Geometry: final body of the model. Coordinates: model frame, mm. A direction names the side the tool comes from. Give positions to 0.01 mm unless a question says otherwise; leave off trailing zeros. Loops run counter-clockwise (first coordinate to the right, second up) from the corner with the lowest first, then second, coordinate; pieces in that order, holes last. Notation, with made-up numbers: (32, 37) - (55, 37) arc R9 ccw to (55, 47) - close; hole circle Ø8 at (-8, 80). An arc over 180 degrees is marked (long way). Use one line per item in the form item = value.
```python
from build123d import *

# Parameters (mm, degrees)
PAD_DEPTH       = 5.3
SKETCH001_R     = 4.15
POCKET_DEPTH    = 2.3
SKETCH002_R     = 2.05
POCKET001_DEPTH = 3.001
FILLET_R        = 2.6
SKETCH003_R     = 1.625
POCKET002_DEPTH = 12.001
FILLET001_R     = 0.9
FILLET002_R     = 5
SKETCH004_R     = 2.05
POCKET003_DEPTH = 5.301
FILLET003_R     = 0.99
CHAMFER_SIZE    = 0.5
SKETCH005_W     = 0.5
SKETCH005_H     = 0.8
POCKET004_DEPTH = 4
CHAMFER001_SIZE = 0.6


with BuildPart() as part:
    # Sketch → Pad (new body)
    with BuildSketch(Plane.XY):
        Polygon((0, 5.5), (-45, 5.5), (-45, -5.5), (0, -5.5), (0, -6.5), (35, -6.5), (35, 6.5), (0, 6.5), align=None)
    extrude(amount=PAD_DEPTH)

    # Sketch001 (on Face10 of Pad) → Pocket (cut)
    with BuildSketch(Plane.XY.offset(5.3)):
        with Locations((-6, 0)):
            Circle(SKETCH001_R)
    extrude(amount=-POCKET_DEPTH, mode=Mode.SUBTRACT)

    # Sketch002 (on Face12 of Pocket) → Pocket001 (cut, through all)
    with BuildSketch(Plane.XY.offset(3)):
        with Locations((-6, 0)):
            Circle(SKETCH002_R)
    extrude(amount=-POCKET001_DEPTH, mode=Mode.SUBTRACT)

    # Fillet
    fillet_edges = [part.edges().sort_by_distance(p)[0] for p in [
        (-45, 0, 5.3),
        (-45, 0, 0),
    ]]
    fillet(fillet_edges, radius=FILLET_R)

    # Sketch003 (on Face1 of Fillet) → Pocket002 (cut, through all)
    with BuildSketch(Plane(origin=(0, 5.5, 0), x_dir=(-1, 0, 0), z_dir=(0, 1, 0))):
        with Locations((42, 2.65)):
            Circle(SKETCH003_R)
    extrude(amount=-POCKET002_DEPTH, mode=Mode.SUBTRACT)

    # Fillet001
    fillet001_edges = [part.edges().sort_by_distance(p)[0] for p in [
        (0, 6.5, 2.65),
        (0, -6.5, 2.65),
    ]]
    fillet(fillet001_edges, radius=FILLET001_R)

    # Fillet002
    fillet002_edges = [part.edges().sort_by_distance(p)[0] for p in [
        (35, 6.5, 2.65),
        (35, -6.5, 2.65),
    ]]
    fillet(fillet002_edges, radius=FILLET002_R)

    # Sketch004 (on Face15 of Fillet002) → Pocket003 (cut, through all)
    with BuildSketch(Plane.XY.offset(5.3)):
        with Locations((-15, 0)):
            Circle(SKETCH004_R)
    extrude(amount=-POCKET003_DEPTH, mode=Mode.SUBTRACT)

    # Fillet003
    fillet003_edges = [part.edges().sort_by_distance(p)[0] for p in [
        (0.263604, -6.236396, 5.3),
        (15.45, -6.5, 5.3),
        (33.535534, -5.035534, 5.3),
        (35, 0, 5.3),
        (33.535534, 5.035534, 5.3),
        (15.45, 6.5, 5.3),
        (0.263604, 6.236396, 5.3),
        (0.263604, 6.236396, 0),
        (15.45, 6.5, 0),
        (33.535534, 5.035534, 0),
        (35, 0, 0),
        (33.535534, -5.035534, 0),
        (15.45, -6.5, 0),
    ]]
    fillet(fillet003_edges, radius=FILLET003_R)

    # Chamfer
    chamfer_edges = [part.edges().sort_by_distance(p)[0] for p in [
        (-17.05, 0, 0),
        (-8.05, 0, 0),
    ]]
    chamfer(chamfer_edges, length=CHAMFER_SIZE)

    # Sketch005 (on Face1 of Chamfer) → Pocket004 (cut)
    with BuildSketch(Plane(origin=(0, 0, 0), x_dir=(1, 0, 0), z_dir=(0, 0, -1))):
        with Locations((-17.15, 0)):
            Rectangle(SKETCH005_W, SKETCH005_H)
    extrude(amount=-POCKET004_DEPTH, mode=Mode.SUBTRACT)

    # Chamfer001
    chamfer001_edges = [part.edges().sort_by_distance(p)[0] for p in [
        (-40.375, 5.5, 2.65),
        (-40.375, -5.5, 2.65),
    ]]
    chamfer(chamfer001_edges, length=CHAMFER001_SIZE)


solid = part.part
```
(1) Cut plane B-B (x = -6). Return the cut outline in (y, z).
Solution:
outline = (-5.5, 0) - (-2.55, 0) - (-2.05, 0.5) - (-2.05, 3) - (-4.15, 3) - (-4.15, 5.3) - (-5.5, 5.3) - close; (2.05, 0.5) - (2.55, 0) - (5.5, 0) - (5.5, 5.3) - (4.15, 5.3) - (4.15, 3) - (2.05, 3) - close
(2) Pin query (flat end, axial travel): P1, Ø2, axis at y = 4.5, z = 3, coming from the +X side; P2, Ø1.6, axis at x = -29, z = 3.5, coming from the -Y side; P3, Ø1, axis at y = -3, z = 4.5, coming from the -X side. Return the tip coordinate at first contact, or that it passes through.
Solution:
P1 = 34.58
P2 = -5.5
P3 = -44.65
(3) Access query for faces 4 (the face through (-5, 2, 3)), 5 (the face through (-5, 5, 5.3)). Directions: +Z, -Z, +X, -X, +Y, -Y. A direction counts if a zero-diameter tool reaches every point of the face in a straight line with its end or side. Return the directions, or none.
Solution:
face_4 = +Z
face_5 = +Z, +X, -X, +Y, -Y
(4) Cut plane A-A (x = -15). Return the cut outline in (y, z).
Solution:
outline = (-5.5, 0) - (-2.55, 0) - (-2.05, 0.5) - (-2.05, 5.3) - (-5.5, 5.3) - close; (2.05, 0.5) - (2.55, 0) - (5.5, 0) - (5.5, 5.3) - (2.05, 5.3) - close
(5) Pull-direction query (X, two-part tool) for faces 1 (the face through (-40.377, 0.069, 2.721)), 2 (the face through (-44.259, -0.077, 4.518)), 3 (the face through (16, 6.5, 3)); classes: released by +X, released by -X, zero draft, split by the parting line, or undercut.
Solution:
face_1 = undercut
face_2 = released by -X
face_3 = zero draft
(6) Cut plane C-C (z = 1.9). Give the number of separate pieces and of enclosed holes in the cut face, plus the area to 3 significant figures.
Solution:
separate_pieces = 2
enclosed_holes = 2
area = 879 mm2
(7) Material intervals for L1, parallel to Y at x = -6, z = 2; L2, parallel to Z at x = -42, y = 2.75 (3 decimals); L3, parallel to X at y = -1, z = 1.6, sorted ascending. Write a range as from..to.
Solution:
L1 = -5.5..-2.05, 2.05..5.5
L2 = 0..1.025, 4.275..5.3
L3 = -44.8..-43.24, -40.76..-16.79, -13.21..-7.79, -4.21..35
